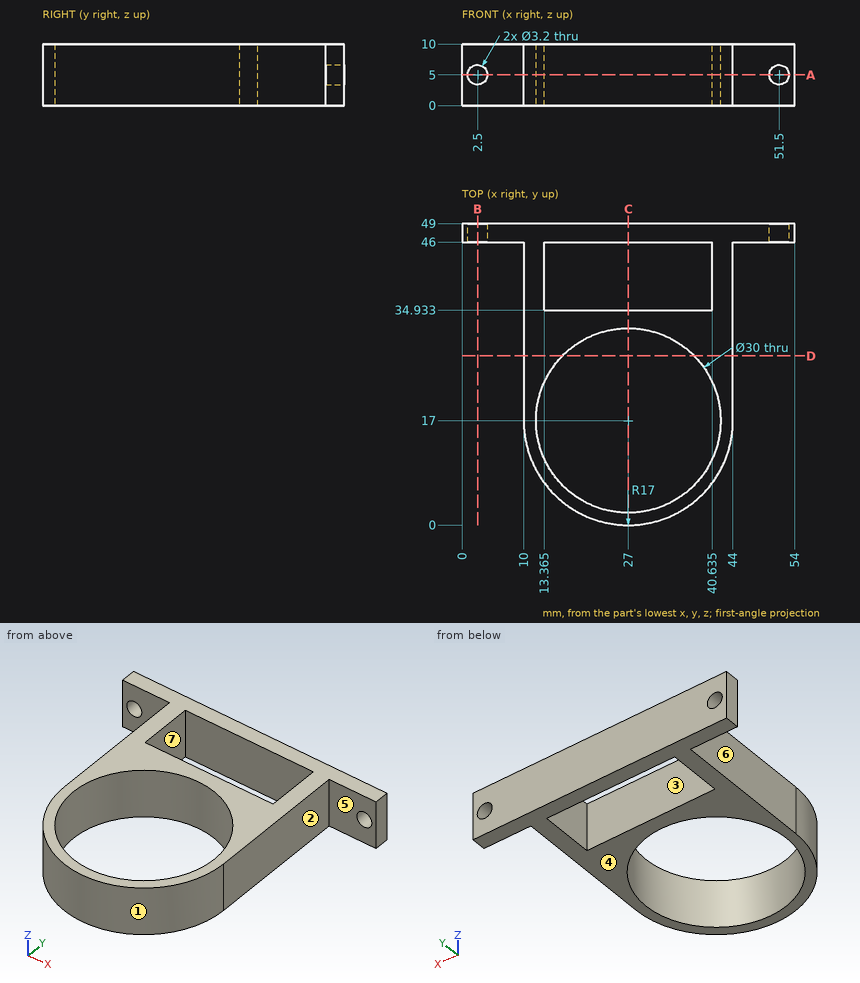
Answer from the drawing. Dimensions are ordinates in mm from the lowest x, y and z of the part. A direction names the side the tool comes from. Round coordinates to 2 decimals unless told otherwise and drop trailing zeros. Write each loop counter-clockwise with the first axis right and the second up, starting at its lowest first coordinate (ties: lowest second). Pieces come first, ordered by that corner, then holes. Notation, with made-up numbers: M 77.25,73 L 97.25,73 A21 cw 97.25,107 Z; hole C 29,60 d10. An arc over 180 degrees is marked long. Write each question's results on one line, items separated by ' | '. Start each with the question number.
Item 1: Which of the six approach directions +Z, -Z, +X, -X, +Y, -Y give full straight-line access (tool end or side, diameter ignored) to the marked faces 5, 6 and 7?
Item 2: Straight lines are drawn through the part: probe 1 along Y at (x, z) = (27, 7); probe 2 along X at (y, z) = (46.8, 5); probe 3 along X at (y, z) = (38, 2) (1 decimal). For each, find the intervals that lie inside material, in ascending order.
Item 3: Given pin 1 Ø2.5 at (x, z) = (2.5, 5) entering from +Y; pin 2 Ø5 at (y, z) = (36.5, 5.5) entering from -X; pin 3 Ø6 at (y, z) = (24.5, 7) entering from +X; pin 4 Ø5 at (x, z) = (19.5, 2) entering from -Y, each flat-ended and moving along its own axis, determine where each tip first touches the part or whether it passes through.
Item 4: Find section A-A on z = 5. Write down the section's boundary in (x, y) (1 decimal), and give its area (3 significant figures).
Item 5: Find section C-C on x = 27. Write down the section's boundary in (y, z).
Item 6: Find section D-D on y = 27.5. Write down the section's boundary in (x, z), and give its area (3 significant figures).
Item 7: The mould has two halves that part along X. Classify the marked faces 1, 2, 3 and 4: +X half, -X half, draft (parallel to the pull), parting line (faces both ways), or undercut.
Item 8: Find section B-B on x = 2.5. Write down the section's boundary in (y, z), and give its area (3 significant figures).
Answer block:
1) face 5: +Z, -Z, +X, -Y | face 6: +Z, -Z, -X, -Y | face 7: +Z, -Z
2) probe 1: y = 0 to 2, 32 to 34.93, 46 to 49 | probe 2: x = 0 to 0.9, 4.1 to 49.9, 53.1 to 54 | probe 3: x = 10 to 13.4, 40.6 to 44
3) pin 1: passes through | pin 2: stops at x = 10 | pin 3: stops at x = 44 | pin 4: stops at y = 0.75
4) outline: M 0,46 L 0.9,46 L 0.9,49 L 0,49 Z; M 4.1,46 L 10,46 L 10,17 A17 ccw 44,17 L 44,46 L 49.9,46 L 49.9,49 L 4.1,49 Z; M 53.1,46 L 54,46 L 54,49 L 53.1,49 Z; hole C 27,17 d30; hole M 13.4,34.9 L 40.6,34.9 L 40.6,46 L 13.4,46 Z | area: 574 mm²
5) outline: M 0,0 L 2,0 L 2,10 L 0,10 Z; M 32,0 L 34.93,0 L 34.93,10 L 32,10 Z; M 46,0 L 49,0 L 49,10 L 46,10 Z
6) outline: M 10,0 L 16.29,0 L 16.29,10 L 10,10 Z; M 37.71,0 L 44,0 L 44,10 L 37.71,10 Z | area: 126 mm²
7) face 1: parting line | face 2: +X half | face 3: undercut | face 4: draft
8) outline: M 46,0 L 49,0 L 49,3.4 L 46,3.4 Z; M 46,6.6 L 49,6.6 L 49,10 L 46,10 Z | area: 20.4 mm²
